from build123d import *

# Parameters (mm, degrees)
ESTRUSIONE_ESTRUSIONE1_DEPTH = 7
SCHIZZO2_R                   = 0.9
TAGLIO_ESTRUSIONE1_DEPTH     = 21.420394218
TAGLIO_ESTRUSIONE2_REACH     = 37.195
SCHIZZO3_R                   = 1.4
SCHIZZO4_W                   = 5.7
SCHIZZO4_H                   = 8
ESTRUSIONE_ESTRUSIONE2_DEPTH = 10.8
SCHIZZO5_W                   = 1.7
SCHIZZO5_H                   = 8
ESTRUSIONE_ESTRUSIONE3_DEPTH = 12
RACCORDO1_R                  = 4
TAGLIO_ESTRUSIONE3_REACH     = 28.169
SCHIZZO6_R                   = 1.5


with BuildPart() as part:
    # Schizzo1 → Estrusione-Estrusione1 (new body)
    with BuildSketch(Plane.XY):
        Polygon((8.3, 11.55), (-4, 11.55), (-4, -11.55), (8.3, -11.55), (8.3, -16.55), (-9.7, -16.55), (-9.7, 16.55), (8.3, 16.55), align=None)
    extrude(amount=ESTRUSIONE_ESTRUSIONE1_DEPTH)

    # Schizzo2 → Taglio-Estrusione1 (cut, through all)
    with BuildSketch(Plane.XY.offset(7)):
        with Locations((2.6, 14.05)):
            Circle(SCHIZZO2_R)
        with Locations(Location((2.6, -14.05, 0), (0, 0, 180))):
            Circle(SCHIZZO2_R)
    extrude(amount=-TAGLIO_ESTRUSIONE1_DEPTH, mode=Mode.SUBTRACT)

    # Schizzo3 → Taglio-Estrusione2 (cut, up to next)
    with BuildSketch(Plane.XZ.offset(16.55), mode=Mode.PRIVATE) as taglio_estrusione2_sk1:
        with Locations(Location((-0.7, 3.5, 0), (0, 0, 270))):
            Circle(SCHIZZO3_R)
    taglio_estrusione2_tool1 = extrude(taglio_estrusione2_sk1.sketch, amount=-TAGLIO_ESTRUSIONE2_REACH, mode=Mode.PRIVATE) & part.part
    add(taglio_estrusione2_tool1.solids().sort_by_distance((-0.7, -16.55, 3.5))[0], mode=Mode.SUBTRACT)

    # Schizzo4 → Estrusione-Estrusione2 (add)
    with BuildSketch(Plane(origin=(0, 0, 0), x_dir=(-1, 0, 0), z_dir=(0, 0, -1))):
        with Locations((6.85, 0)):
            Rectangle(SCHIZZO4_W, SCHIZZO4_H)
    extrude(amount=ESTRUSIONE_ESTRUSIONE2_DEPTH)

    # Schizzo5 → Estrusione-Estrusione3 (add)
    with BuildSketch(Plane(origin=(-4, 0, 0), x_dir=(0, 0, -1), z_dir=(1, 0, 0))):
        with Locations((9.95, 0)):
            Rectangle(SCHIZZO5_W, SCHIZZO5_H)
    extrude(amount=ESTRUSIONE_ESTRUSIONE3_DEPTH)

    # Raccordo1
    raccordo1_edges = [part.edges().sort_by_distance(p)[0] for p in [
        (8, 4, -9.95),
        (8, -4, -9.95),
    ]]
    fillet(raccordo1_edges, radius=RACCORDO1_R - 0.0001)  # a hair under: the kernel refuses the full size

    # Schizzo6 → Taglio-Estrusione3 (cut, up to next)
    with BuildSketch(Plane(origin=(0, 0, -10.8), x_dir=(-1, 0, 0), z_dir=(0, 0, -1)), mode=Mode.PRIVATE) as taglio_estrusione3_sk1:
        with Locations((-2.6, 0)):
            Circle(SCHIZZO6_R)
    taglio_estrusione3_tool1 = extrude(taglio_estrusione3_sk1.sketch, amount=-TAGLIO_ESTRUSIONE3_REACH, mode=Mode.PRIVATE) & part.part
    add(taglio_estrusione3_tool1.solids().sort_by_distance((2.6, 0, -10.8))[0], mode=Mode.SUBTRACT)


solid = part.part
Can you work these out from the model? Positions are in its coordinate system, mm. A direction names the side the tool comes from. Give positions to 0.01 mm unless a question says otherwise; leave off trailing zeros. Order: outer loops, then holes, each group sorted by start corner. A loop starts at its lowest first (then second) coordinate and runs counter-clockwise, first axis right, second up. Notation, with made-up numbers: M -38,-25.5 L 0,-25.5 A24 ccw 0,5.5 Z; hole C 46.25,41 d2. An arc over 180 degrees is marked long. One line per item, written item: value.
Item 1: If we section it at B-B on z = 3.5: Write out the boundary of the cut face in (x, y).
Verdict:
outline: M -9.7,-16.55 L -2.1,-16.55 L -2.1,-11.55 L -4,-11.55 L -4,11.55 L 8.3,11.55 L 8.3,16.55 L -9.7,16.55 Z; M 0.7,-16.55 L 8.3,-16.55 L 8.3,-11.55 L 0.7,-11.55 Z; hole C 2.6,-14.05 d1.8; hole C 2.6,14.05 d1.8
Item 2: Please list where these lines run through material, in increasing order: line 1 (Y direction, x = 2.6, z = 4); line 2 (X direction, y = -15, z = 3.5); line 3 (Y direction, x = 5.5, z = 3).
Verdict:
line 1: -16.55 to -14.95, -13.15 to -11.55, 11.55 to 13.15, 14.95 to 16.55
line 2: -9.7 to -2.1, 0.7 to 8.3
line 3: -16.55 to -11.55, 11.55 to 16.55
Item 3: For faces 1 (the face through (-3, -12, 0)), 2 (the face through (-1.24, -14.08, 2.21)), 3 (the face through (-4, 0, 1)), 4 (the face through (0.6, -0.1, -9.1)), which set-ups out of +Z, -Z, +X, -X, +Y, -Y let a thin tool reach every point of the face, with its end or its side?
Verdict:
face 1: -Z, +X, -X, -Y
face 2: -Y
face 3: +Z, +X
face 4: +Z, +X, +Y, -Y
Item 4: If we mould it in two halves opening along Y, with no side actions, what happens to faces 5 (the face through (2, 11.55, 3)), 6 (the face through (-3, 12, 0)), 7 (the face through (-6, -4, -5)), 8 (the face through (6.859, 2.797, -9.962))? For each: pulls with the +Y half, pulls with the -Y half, needs draft (parallel to the pull), parting line crosses it, or undercut.
Verdict:
face 5: undercut
face 6: needs draft
face 7: pulls with the -Y half
face 8: pulls with the +Y half
Item 5: If we section it at A-A on y = -14.05: Write out the boundary of the cut face in (x, z), and give its area (3 significant figures).
Verdict:
outline: M -9.7,0 L 1.7,0 L 1.7,7 L -9.7,7 Z; M 3.5,0 L 8.3,0 L 8.3,7 L 3.5,7 Z; hole C -0.7,3.5 d2.8
area: 107 mm2
Item 6: For pin 1 (5 mm diameter, centred on x = 0, y = 11.5, fed in from -Z); pin 2 (1.4 mm diameter, centred on x = 2.6, y = -14.05, fed in from -Z); pin 3 (6.5 mm diameter, centred on x = 2.5, y = 0, fed in from +Z); pin 4 (5.5 mm diameter, centred on x = -1.5, z = -3, fed in from +Y), each with a flat end and sliding along its axis, tell me the tip position at first contact or that it passes through.
Verdict:
pin 1: z = 0
pin 2: through
pin 3: z = -9.1
pin 4: y = 4
Item 7: If we section it at C-C on y = 14.05: Write out the boundary of the cut face in (x, z), and give its area (3 significant figures).
Verdict:
outline: M -9.7,0 L 1.7,0 L 1.7,7 L -9.7,7 Z; M 3.5,0 L 8.3,0 L 8.3,7 L 3.5,7 Z
area: 113 mm2
